```python
from build123d import *

# Parameters (mm, degrees)
SKETCH1_R           = 2.5
BOSS_EXTRUDE1_DEPTH = 7
SKETCH3_W           = 0.625
SKETCH3_H           = 0.5


with BuildPart() as part:
    # Sketch1 → Boss-Extrude1 (new body)
    with BuildSketch(Plane(origin=(0, 0, 0), x_dir=(1, 0, 0), z_dir=(0, 1, 0))):
        with Locations(Location((0, 0, 0), (0, 0, 270))):
            Circle(SKETCH1_R)
    extrude(amount=BOSS_EXTRUDE1_DEPTH)

    # Sketch2 → Revolve1 (revolve)
    with BuildSketch(Plane.XY):
        with BuildLine():
            Line((0, 7), (3, 7))
            ThreePointArc((3, 7), (2.121320344, 9.121320344), (0, 10))
            Line((0, 10), (0, 7))
        make_face()
    revolve(axis=Axis((0, 7, 0), (0, 1, 0)))

    # Sketch3 → Cut-Revolve1 (revolve, cut)
    with BuildSketch(Plane.XY, mode=Mode.PRIVATE) as cut_revolve1_sk:
        with Locations((2.1875, 0.75)):
            Rectangle(SKETCH3_W, SKETCH3_H)
    revolve(cut_revolve1_sk.sketch.rotate(Axis((0, 7, 0), (0, -1, 0)), 180), axis=Axis((0, 7, 0), (0, -1, 0)), mode=Mode.SUBTRACT)


solid = part.part
```
Work out the finished part from the listing and answer in its coordinate system (mm). A direction names the side the tool comes from. Round coordinates to 2 decimals unless told otherwise and drop trailing zeros. Write each loop counter-clockwise with the first axis right and the second up, starting at its lowest first coordinate (ties: lowest second). Pieces come first, ordered by that corner, then holes. Notation, with made-up numbers: (63.5, -19) - (108.5, -19) arc R10 ccw to (108.5, -2) - close; hole circle Ø10 at (-9, -28.75). An arc over 180 degrees is marked (long way). Return JSON: item names as keys, results as strings. Group by question number.
Q1. The part is cut by section C-C on z = 0. Write down the section's boundary in (x, y) (3 decimals), then the cut area to 3 significant figures.
Q2. Find the intervals of material crossed by L1, parallel to Y at x = 0.45, z = 2.1; L2, parallel to Z at x = 0.1, y = 1.5; L3, parallel to Y at x = -0.35, z = -2.7, in increasing order.
Q3. The part is cut by section D-D on z = 2.35. Write down the section's boundary in (x, y), then the cut area to 3 significant figures.
Q4. For faces 1 (the flat face through (1, 1, -2)), 2 (the flat face through (2, 7, -2)), determine the directions among +Z, -Z, +X, -X, +Y, -Y from which every point of the face is accessible in a straight line to the end or side of a thin tool.
Q5. The part is cut by section A-A on x = 2.2. Write down the section's boundary in (y, z).
Q6. Each of these flat-tipped pins is pushed along its axis until it touches: pin 1 Ø2 at (x, z) = (1.5, 0) entering from -Y; pin 2 Ø2 at (x, y) = (1, 3) entering from -Z; pin 3 Ø1 at (y, z) = (1.5, 2) entering from +X; pin 4 Ø1 at (x, y) = (2.5, 6) entering from +Z. Where does it stop, or does it pass through?
Q7. The mould has two halves that part along Y. Classify faces 3 (the flat face through (1, 0.5, -2)), 4 (the flat face through (0, 0, 0)), 5 (the cylindrical face through (-1.01, 0.75, -1.58)), 6 (the cylindrical face through (-2.44, 0.25, -0.54)): released by +Y, released by -Y, zero draft, split by the parting line, or undercut.
Q8. The part is cut by section B-B on x = 0. Write down the section's boundary in (y, z) (3 decimals), then the cut area to 3 significant figures.
Solved:
{
 "1": {"outline": "(-3, 7) - (-2.5, 7) - (-2.5, 1) - (-1.875, 1) - (-1.875, 0.5) - (-2.5, 0.5) - (-2.5, 0) - (2.5, 0) - (2.5, 0.5) - (1.875, 0.5) - (1.875, 1) - (2.5, 1) - (2.5, 7) - (3, 7) arc R3 ccw to start", "area": "48.5 mm²"},
 "2": {"L1": "0 to 0.5, 1 to 9.09", "L2": "-2.5 to 2.5", "L3": "7 to 8.26"},
 "3": {"outline": "(-1.86, 7) - (-0.85, 7) - (-0.85, 1) - (0.85, 1) - (0.85, 7) - (1.86, 7) arc R1.86 ccw to start; (-0.85, 0) - (0.85, 0) - (0.85, 0.5) - (-0.85, 0.5) - close", "area": "16.6 mm²"},
 "4": {"face 1": "none", "face 2": "-Y"},
 "5": {"outline": "(0, -1.19) - (0.5, -1.19) - (0.5, 1.19) - (0, 1.19) - close; (1, -1.19) - (7, -1.19) - (7, -2.04) arc R2.04 ccw to (7, 2.04) - (7, 1.19) - (1, 1.19) - close"},
 "6": {"pin 1": "y = 0", "pin 2": "z = -2.5", "pin 3": "x = 2", "pin 4": "z = 1.5"},
 "7": {"face 3": "undercut", "face 4": "released by -Y", "face 5": "undercut", "face 6": "zero draft"},
 "8": {"outline": "(0, -2.5) - (0.5, -2.5) - (0.5, -1.875) - (1, -1.875) - (1, -2.5) - (7, -2.5) - (7, -3) arc R3 ccw to (7, 3) - (7, 2.5) - (1, 2.5) - (1, 1.875) - (0.5, 1.875) - (0.5, 2.5) - (0, 2.5) - close", "area": "48.5 mm²"}
}
